Part model, mm, in its own coordinate system. Face numbers are marked on the shaded views. A direction names the side the tool comes from. Coordinates: 2 decimals unless noted, no trailing zeros. Loops run counter-clockwise (first coordinate to the right, second up) from the corner with the lowest first, then second, coordinate; pieces in that order, holes last. Notation, with made-up numbers: M -19,87.25 L 28,87.25 A20 cw 28,124.25 Z; hole C 43.25,84.5 d9. An arc over 180 degrees is marked long. Answer as a JSON object with one key per item and string values. Group by question number.
1. Drill centre lines: L1, parallel to Y at x = 1.3, z = 63.5; L2, parallel to Y at x = 9.25, z = 33.5 (3 decimals); L3, parallel to X at y = 36.5, z = 132.5 (3 decimals). Where is each one in solid material? Low to high.
2. Saw through at B-B on x = 18. Write the cut outline in (y, z) (3 decimals), then the cut area to 3 significant figures.
3. 3-axis set-ups, long thin cutter, end or side, ignore diameter. For the marked faces 4 and 5: which of +Z, -Z, +X, -X, +Y, -Y reach the whole face in a straight line?
4. Saw through at A-A on z = 127. Count the separate pieces of the cut face and the enclosed holes in it, then the cut area to 3 significant figures.
5. Drop flat-ended pins along their axis: pin 1 Ø12 at (y, z) = (20, 105) entering from -X; pin 2 Ø10 at (x, y) = (13, 18.5) entering from -Z. Give the stop position or say it passes through.
6. Saw through at D-D on z = 48.5. Write the cut outline in (x, y) (3 decimals), then the cut area to 3 significant figures.
7. Mould opens along Y. For the marked faces 1, 2 and 3 say: released by +Y, released by -Y, zero draft, split by the parting line, or undercut.
8. Saw through at C-C on y = 20. Write the cut outline in (x, z) (3 decimals).
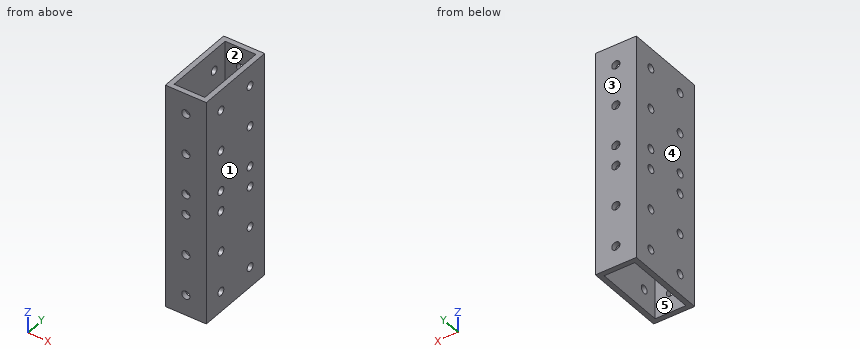
Autodesk Inventor part; units mm, degrees
ref_plane "YZ Plane" through (0, 0, 0) normal (1, 0, 0) x (0, 1, 0)
ref_plane "XZ Plane" through (0, 0, 0) normal (0, 1, 0) x (-1, 0, 0)
ref_plane "XY Plane" through (0, 0, 0) normal (0, 0, 1) x (1, 0, 0)
sketch "Sketch1" plane through (0, 0, 0) normal (0, 0, 1) x (1, 0, 0)
  line L0 (0, 0) -> (25.4, 0)
  line L1 (25.4, 0) -> (25.4, 50.8)
  line L2 (25.4, 50.8) -> (0, 50.8)
  line L3 (0, 50.8) -> (0, 0)
  line L4 (3.175, 3.175) -> (22.225, 3.175)
  line L5 (22.225, 3.175) -> (22.225, 47.625)
  line L6 (22.225, 47.625) -> (3.175, 47.625)
  line L7 (3.175, 47.625) -> (3.175, 3.175)
  dimension "d0" = 25.4
  dimension "d1" = 50.8
  dimension "d2" = 3.175
  dimension "d3" = 3.175
  dimension "d4" = 3.175
  dimension "d5" = 3.175
extrude "Extrusion1" add sketch "Sketch1" along normal blind 139.7
sketch "Sketch2" plane through (25.4, 0, 0) normal (1, 0, 0) x (0, 0, -1)
  line L0 (0, 0) -> (0, 50.8)
  line L1 (0, 0) -> (0, 12.7)
  line L2 (0, 12.7) -> (-139.7, 12.7)
  line L3 (-139.7, 47.625) -> (-139.7, 3.175)
  line L4 (-139.7, 0) -> (-139.7, 50.8)
  line L5 (-139.7, 50.8) -> (-139.7, 38.1)
  line L6 (-139.7, 38.1) -> (0, 38.1)
  line L7 (-139.7, 38.1) -> (-127, 38.1)
  line L8 (-127, 38.1) -> (-127, 12.7)
  line L9 (0, 38.1) -> (-12.7, 38.1)
  line L10 (-12.7, 38.1) -> (-12.7, 12.7)
  line L11 (-12.7, 38.1) -> (-38.1, 38.1)
  line L12 (-38.1, 38.1) -> (-63.5, 38.1)
  line L13 (-127, 38.1) -> (-101.6, 38.1)
  line L14 (-101.6, 38.1) -> (-76.2, 38.1)
  circle A0 centre (-127, 38.1) radius 2.54
  circle A1 centre (-127, 12.7) radius 2.54
  circle A2 centre (-101.6, 38.1) radius 2.54
  circle A3 centre (-76.2, 38.1) radius 2.54
  circle A4 centre (-63.5, 38.1) radius 2.54
  circle A5 centre (-38.1, 38.1) radius 2.54
  circle A6 centre (-12.7, 38.1) radius 2.54
  circle A7 centre (-12.7, 12.7) radius 2.54
  circle A8 centre (-38.1, 12.7) radius 2.54
  circle A9 centre (-63.5, 12.7) radius 2.54
  circle A10 centre (-76.2, 12.7) radius 2.54
  circle A11 centre (-101.6, 12.7) radius 2.54
  dimension "d8" = 12.7
  dimension "d9" = 12.7
  dimension "d10" = 12.7
  dimension "d11" = 12.7
  dimension "d12" = 25.4
  dimension "d13" = 25.4
  dimension "d14" = 25.4
  dimension "d15" = 25.4
  dimension "d16" = 5.08
extrude "Extrusion2" cut sketch "Sketch2" against normal blind 25.4 contours A7 L2 | L2 L10 A7 | A6 L10 L6 | L6 A6 | L2 A7 L10 | L10 A6 L6 | A8 L2 | L2 A8 | A5 L6 | L6 A5 | A9 L2 | L2 A9 | A4 L6 | L6 A4 | A10 L2 | L2 A10 | A3 L6 | L6 A3 | A11 L2 | L2 A11 | A2 L6 | L6 A2 | A1 L2 | L2 L8 A1 | A0 L8 L6 | L6 A0 | L2 A1 L8 | L8 A0 L6
sketch "Sketch3" plane through (0, 50.8, 0) normal (0, 1, 0) x (1, 0, 0)
  line L0 (3.175, 0) -> (22.225, 0)
  line L1 (12.7, 0) -> (12.7, -139.7)
  line L2 (12.7, -139.7) -> (12.7, -127)
  line L3 (12.7, -127) -> (12.7, -101.6)
  line L4 (12.7, -101.6) -> (12.7, -76.2)
  line L5 (12.7, 0) -> (12.7, -12.7)
  line L6 (12.7, -12.7) -> (12.7, -38.1)
  line L7 (12.7, -38.1) -> (12.7, -63.5)
  circle A0 centre (12.7, -12.7) radius 2.54
  circle A1 centre (12.7, -38.1) radius 2.54
  circle A2 centre (12.7, -63.5) radius 2.54
  circle A3 centre (12.7, -76.2) radius 2.54
  circle A4 centre (12.7, -101.6) radius 2.54
  circle A5 centre (12.7, -127) radius 2.54
  point P0 (0, 0)
  dimension "d19" = 12.7
  dimension "d20" = 25.4
  dimension "d21" = 25.4
  dimension "d22" = 12.7
  dimension "d23" = 25.4
  dimension "d24" = 25.4
  dimension "d25" = 5.08
extrude "Extrusion3" cut sketch "Sketch3" against normal blind 111.125
properties part number "5.5 2x2" material "Aluminum 6061"
Outcome:
{
 "1": {"L1": "y = 0 to 10.16, 15.24 to 35.56, 40.64 to 50.8", "L2": "y = 0 to 3.175, 47.625 to 50.8", "L3": "x = 0 to 3.175, 22.225 to 25.4"},
 "2": {"outline": "M 0,0 L 3.175,0 L 3.175,139.7 L 0,139.7 Z; M 47.625,0 L 50.8,0 L 50.8,139.7 L 47.625,139.7 Z", "area": "887 mm²"},
 "3": {"face 4": "+Z, -Z, -X, +Y, -Y", "face 5": "+Z, -Z"},
 "4": {"separate pieces": "6", "enclosed holes": "0", "area": "347 mm²"},
 "5": {"pin 1": "stops at x = 0", "pin 2": "passes through"},
 "6": {"outline": "M 0,0 L 25.4,0 L 25.4,50.8 L 0,50.8 Z; hole M 3.175,3.175 L 22.225,3.175 L 22.225,47.625 L 3.175,47.625 Z", "area": "444 mm²"},
 "7": {"face 1": "zero draft", "face 2": "undercut", "face 3": "released by +Y"},
 "8": {"outline": "M 0,0 L 3.175,0 L 3.175,139.7 L 0,139.7 Z; M 22.225,0 L 25.4,0 L 25.4,139.7 L 22.225,139.7 Z"}
}
